```python
from build123d import *

# Parameters (mm, degrees)
EXTRUDE_1285_DEPTH = 17
EXTRUDE_1381_DEPTH = 1


with BuildPart() as part:
    # Sketch 270 → Extrude 1285 (new body)
    with BuildSketch(Plane.XY):
        Polygon((5.35, 13.15), (5.35, 2), (0, 2), (0, 0), (30, 0), (30, 2), (24.65, 2), (24.65, 9.946320344), (21.446320344, 13.15), (17.825, 13.15), (17.825, 11.65), (20.825, 11.65), (23.15, 9.325), (23.15, 5.825), (20.825, 3.5), (6.85, 3.5), (6.85, 11.65), (9.85, 11.65), (9.85, 13.15), align=None)
    extrude(amount=EXTRUDE_1285_DEPTH)

    # Sketch 1_6 → Extrude 1381 (add)
    with BuildSketch(Plane.XY):
        Polygon((17.825, 11.65), (20.825, 11.65), (23.15, 9.325), (23.15, 5.825), (20.825, 3.5), (6.85, 3.5), (6.85, 11.65), (9.85, 11.65), (9.85, 10.9), (7.6, 10.9), (7.6, 4.25), (20.514339828, 4.25), (22.4, 6.135660172), (22.4, 9.014339828), (20.514339828, 10.9), (17.825, 10.9), align=None)
    extrude(amount=EXTRUDE_1381_DEPTH)


solid = part.part
```
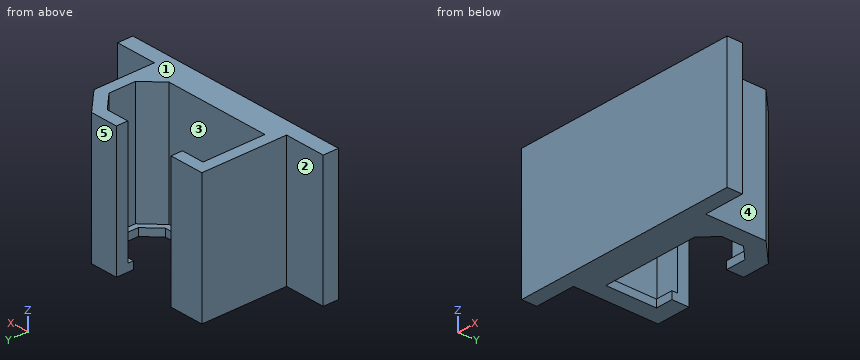
Input: part model. Units: mm. Frame: model coordinates. Face numbers are marked on the shaded views. A direction names the side the tool comes from. Round coordinates to 2 decimals unless told otherwise and drop trailing zeros. Loops run counter-clockwise (first coordinate to the right, second up) from the corner with the lowest first, then second, coordinate; pieces in that order, holes last. Notation, with made-up numbers: M 63,-15 L 108,-15 A27 cw 108,21 Z; hole C 80.25,4 d5. An arc over 180 degrees is marked long. Answer in a Markdown table with one row per item. Add a question column.
1. Section D-D (x = 3.5). Output: boundary loops of the cut face in (y, z), and give its area (3 significant figures).
2. Contact query for flat-ended pins moving along their axis: pin 1 (2.5 mm diameter, centred on y = 7.5, z = 11, fed in from +X); pin 2 (2.5 mm diameter, centred on x = 27, z = 4.5, fed in from +Y); pin 3 (3 mm diameter, centred on x = 25, z = 6.5, fed in from +Y). Output: stop coordinate, or through.
3. Section C-C (z = 4.5). Output: boundary loops of the cut face in (x, y) (3 decimals), and give its area (3 significant figures).
4. Ray query, probe 1 along X at (y, z) = (9, 6); probe 2 along Y at (x, z) = (9.25, 10.5); probe 3 along Y at (x, z) = (2.75, 2.75). Return the intervals inside material, ascending.
5. Set-up query: the marked faces 1, 2, 3, 4 and 5. Return all of +Z, -Z, +X, -X, +Y, -Y with unobstructed straight access to the full face (end or side cutting, diameter ignored); none if empty.
6. Section B-B (y = 7.5). Output: boundary loops of the cut face in (x, z), and give its area (3 significant figures).
7. Section A-A (x = 18.5). Output: boundary loops of the cut face in (y, z).
Values follow:
| question | item | result |
|---|---|---|
| 1 | outline | M 0,0 L 2,0 L 2,17 L 0,17 Z |
| 1 | area | 34.0 mm^2 |
| 2 | pin 1 | x = 24.65 |
| 2 | pin 2 | y = 2 |
| 2 | pin 3 | y = 11.1 |
| 3 | outline | M 0,0 L 30,0 L 30,2 L 24.65,2 L 24.65,9.946 L 21.446,13.15 L 17.825,13.15 L 17.825,11.65 L 20.825,11.65 L 23.15,9.325 L 23.15,5.825 L 20.825,3.5 L 6.85,3.5 L 6.85,11.65 L 9.85,11.65 L 9.85,13.15 L 5.35,13.15 L 5.35,2 L 0,2 Z |
| 3 | area | 131 mm^2 |
| 4 | probe 1 | 5.35 to 6.85, 23.15 to 24.65 |
| 4 | probe 2 | 0 to 3.5, 11.65 to 13.15 |
| 4 | probe 3 | 0 to 2 |
| 5 | face 1 | +Z, +X, -X, +Y, -Y |
| 5 | face 2 | +Z, -Z, -X, +Y |
| 5 | face 3 | +Z |
| 5 | face 4 | +Z, -Z, +X, +Y |
| 5 | face 5 | +Z, -Z, +X, -X, +Y |
| 6 | outline | M 5.35,0 L 7.6,0 L 7.6,1 L 6.85,1 L 6.85,17 L 5.35,17 Z; M 22.4,0 L 24.65,0 L 24.65,17 L 23.15,17 L 23.15,1 L 22.4,1 Z |
| 6 | area | 52.5 mm^2 |
| 7 | outline | M 0,0 L 4.25,0 L 4.25,1 L 3.5,1 L 3.5,17 L 0,17 Z; M 10.9,0 L 13.15,0 L 13.15,17 L 11.65,17 L 11.65,1 L 10.9,1 Z |
